The model under review builds one solid part; all positions refer to its coordinate system, in mm. A direction names the side the tool comes from. Round coordinates to 2 decimals unless told otherwise and drop trailing zeros. Write each loop counter-clockwise with the first axis right and the second up, starting at its lowest first coordinate (ties: lowest second). Pieces come first, ordered by that corner, then holes. Notation, with made-up numbers: (19, 23.25) -> (74, 23.25) arc R29 ccw to (74, 52.25) -> close; hole circle Ø10 at (84.25, 52.25). An arc over 180 degrees is marked (long way). Answer in a Markdown table with one row per item. Add a question column.
```python
from build123d import *

# Parameters (mm, degrees)
EXTRUDE_1_DEPTH      = 20
EXTRUDE_1_DEPTH_BACK = 20
SKETCH_1_W           = 10
SKETCH_1_H           = 35
FILLET_1_R           = 20
SKETCH_2_R           = 5.5
CUT_EXTRUDE_1_DEPTH  = 49.79805324
EXTRUDE_2_DEPTH      = 5
EXTRUDE_2_DEPTH_BACK = 5
SKETCH_3_R           = 3.5
CUT_EXTRUDE_2_DEPTH  = 51.249378106
SKETCH_4_R           = 6.5
CUT_EXTRUDE_3_DEPTH  = 5


with BuildPart() as part:
    # Эскиз1 → Бобышка-Вытянуть1 (new, two sides: drawn at the far end of the back side and taken through both)
    with BuildSketch(Plane(origin=(0, 0, 0), x_dir=(0, 0, -1), z_dir=(1, 0, 0)).offset(-EXTRUDE_1_DEPTH_BACK)):
        Rectangle(SKETCH_1_W, SKETCH_1_H)
        Polygon((-5, -17.5), (-14, -17.5), (-30, -17.5), (-30, -27.5), (30, -27.5), (30, -17.5), (14, -17.5), (5, -17.5), align=None)
    extrude(amount=EXTRUDE_1_DEPTH + EXTRUDE_1_DEPTH_BACK)

    # Скругление1
    fillet_1_edges = [part.edges().sort_by_distance(p)[0] for p in [
        (-20, 17.5, 0),
        (20, 17.5, 0),
    ]]
    fillet(fillet_1_edges, radius=FILLET_1_R - 0.0001)  # a hair under: the kernel refuses the full size

    # Эскиз2 → Вырез-Вытянуть1 (cut, through all)
    with BuildSketch(Plane.XY.offset(5)):
        with Locations((0, -2.5)):
            Circle(SKETCH_2_R)
    extrude(amount=-CUT_EXTRUDE_1_DEPTH, mode=Mode.SUBTRACT)

    # Эскиз1<3> → Бобышка-Вытянуть2 (add, two sides: drawn at the far end of the back side and taken through both)
    with BuildSketch(Plane(origin=(0, 0, 0), x_dir=(0, 0, -1), z_dir=(1, 0, 0)).offset(-EXTRUDE_2_DEPTH_BACK)):
        Polygon((-5, -9.5), (-14, -17.5), (-5, -17.5), align=None)
        Polygon((5, -9.5), (5, -17.5), (14, -17.5), align=None)
    extrude(amount=EXTRUDE_2_DEPTH + EXTRUDE_2_DEPTH_BACK)

    # Эскиз3 → Вырез-Вытянуть2 (cut, through all)
    with BuildSketch(Plane(origin=(0, -17.5, 0), x_dir=(1, 0, 0), z_dir=(0, 1, 0))):
        with Locations(Location((-12, -22, 0), (0, 0, 270))):
            Circle(SKETCH_3_R)
        with Locations(Location((12, 22, 0), (0, 0, 270))):
            Circle(SKETCH_3_R)
    extrude(amount=-CUT_EXTRUDE_2_DEPTH, mode=Mode.SUBTRACT)

    # Эскиз4 → Вырез-Вытянуть3 (cut)
    with BuildSketch(Plane(origin=(0, -17.5, 0), x_dir=(1, 0, 0), z_dir=(0, 1, 0))):
        with Locations(Location((12, 22, 0), (0, 0, 270))):
            Circle(SKETCH_4_R)
    extrude(amount=-CUT_EXTRUDE_3_DEPTH, mode=Mode.SUBTRACT)


solid = part.part
```
1. Add section B-B on x = 14. Write out the cut boundary in (y, z), plus the area to 3 significant figures.
2. Mouldability with a two-part tool opening along Z and no side actions: class faces 5 (the flat face through (0, -17.5, -18)), 6 (the flat face through (0, -23, -30)), 7 (the flat face through (9, -22.5, -19)) as pulls with the +Z half, pulls with the -Z half, needs draft (parallel to the pull), parting line crosses it, or undercut.
3. Add section A-A on z = 22. Write out the cut boundary in (x, y), plus the area to 3 significant figures.
4. Add section C-C on y = 0.5. Write out the cut boundary in (x, z).
5. Tool access review of faces 1 (the flat face through (-5, -15, 8)), 2 (the flat face through (-5, -15, -7)), 3 (the flat face through (0, -17.5, 17)), 4 (the cylindrical face through (12.286, -19.965, -28.494)): name each direction out of +Z, -Z, +X, -X, +Y, -Y from which nothing blocks a thin tool from reaching the whole face with its end or side.
6. For L1, parallel to X at y = -25.6, z = -22; L2, parallel to Y at x = 0, z = -25; L3, parallel to Y at x = 8.5, z = -18, list the stretches that pass through material, from the lowest coordinate up.
7. Insertion check: pin 1 Ø9 at (x, y) = (0, -2.5) entering from -Z; pin 2 Ø7.5 at (x, z) = (-8.5, 20.5) entering from +Y; pin 3 Ø3 at (x, y) = (12.5, 3) entering from -Z; pin 4 Ø12 at (x, y) = (-7.5, -10) entering from +Z. Each pin has a flat end and moves straight along its axis. Give the tip position at first contact, or say it passes through.
8. Add section D-D on z = -22. Write out the cut boundary in (x, y).
Filled in:
| question | item | result |
|---|---|---|
| 1 | outline | (-27.5, -30) -> (-17.5, -30) -> (-17.5, -28.18) -> (-22.5, -28.18) -> (-22.5, -24.87) -> (-27.5, -24.87) -> close; (-27.5, -19.13) -> (-22.5, -19.13) -> (-22.5, -15.82) -> (-17.5, -15.82) -> (-17.5, -5) -> (11.78, -5) -> (11.78, 5) -> (-17.5, 5) -> (-17.5, 30) -> (-27.5, 30) -> close |
| 1 | area | 802 mm² |
| 2 | face 5 | needs draft |
| 2 | face 6 | pulls with the -Z half |
| 2 | face 7 | undercut |
| 3 | outline | (-20, -27.5) -> (-15.5, -27.5) -> (-15.5, -17.5) -> (-20, -17.5) -> close; (-8.5, -27.5) -> (20, -27.5) -> (20, -17.5) -> (-8.5, -17.5) -> close |
| 3 | area | 330 mm² |
| 4 | outline | (-19.77, -5) -> (-4.61, -5) -> (-4.61, 5) -> (-19.77, 5) -> close; (4.61, -5) -> (19.77, -5) -> (19.77, 5) -> (4.61, 5) -> close |
| 5 | face 1 | +Z, -X, +Y |
| 5 | face 2 | -Z, -X, +Y |
| 5 | face 3 | +Z, +Y |
| 5 | face 4 | +Y |
| 6 | L1 | -20 to 8.5, 15.5 to 20 |
| 6 | L2 | -27.5 to -17.5 |
| 6 | L3 | -27.5 to -22.5 |
| 7 | pin 1 | through |
| 7 | pin 2 | y = -17.5 |
| 7 | pin 3 | z = -5 |
| 7 | pin 4 | z = 11.7 |
| 8 | outline | (-20, -27.5) -> (8.5, -27.5) -> (8.5, -22.5) -> (5.5, -22.5) -> (5.5, -17.5) -> (-20, -17.5) -> close; (15.5, -27.5) -> (20, -27.5) -> (20, -17.5) -> (18.5, -17.5) -> (18.5, -22.5) -> (15.5, -22.5) -> close |
